For this review, take the finished solid that the model builds, in its own axes (mm). A direction names the side the tool comes from. Give positions to 0.01 mm unless a question says otherwise; leave off trailing zeros. Loops run counter-clockwise (first coordinate to the right, second up) from the corner with the lowest first, then second, coordinate; pieces in that order, holes last. Notation, with made-up numbers: (-34.5, -18) - (23.5, -18) arc R26 ccw to (23.5, 15) - close; hole circle Ø3 at (56.25, 6). An arc over 180 degrees is marked (long way). Answer as CSV lines item,"result".
from build123d import *


with BuildPart() as f2:
    # F2: sweep along a path in F1
    with BuildLine(Plane.XY) as f2_path:
        Line((0, 717.2), (0, 6))
        Line((0, 6), (1631.95, 6))
        Line((1631.95, 6), (1631.95, 717.2))
        Line((1631.95, 717.2), (0, 717.2))
    # F0 (on Right) → F2 (sweep)
    with BuildSketch(Plane.YZ):
        with BuildLine():
            Line((0, -6), (0, -70.7))
            Line((0, -70.7), (6, -70.7))
            Line((6, -70.7), (6, -68))
            Line((6, -68), (4.8, -68))
            Line((4.8, -68), (4.8, -69.5))
            Line((4.8, -69.5), (1.5, -69.5))
            Line((1.5, -69.5), (1.5, -6))
            ThreePointArc((1.5, -6), (2.8180194847, -2.8180194847), (6, -1.5))
            Line((6, -1.5), (8.6, -1.5))
            Line((8.6, -1.5), (8.6, -9.4503759398))
            Line((8.6, -9.4503759398), (6, -12.5))
            Line((6, -12.5), (6, -13.7))
            Line((6, -13.7), (6.5538461538, -13.7))
            Line((6.5538461538, -13.7), (8.6, -11.3))
            Line((8.6, -11.3), (8.6, -13.7))
            Line((8.6, -13.7), (43.1, -13.7))
            Line((43.1, -13.7), (43.1, -12.5))
            Line((43.1, -12.5), (9.8, -12.5))
            Line((9.8, -12.5), (9.8, -4.5))
            Line((9.8, -4.5), (13.5, -4.5))
            Line((13.5, -4.5), (13.5, -3.3))
            Line((13.5, -3.3), (9.8, -3.3))
            Line((9.8, -3.3), (9.8, -1.5))
            Line((9.8, -1.5), (12.2, -1.5))
            Line((12.2, -1.5), (12.2, 0))
            Line((12.2, 0), (6, 0))
            ThreePointArc((6, 0), (1.7573593129, -1.7573593129), (0, -6))
        make_face()
    sweep(path=f2_path.line, transition=Transition.RIGHT)


solid = f2.part
1) Draft analysis for pull direction Z (two halves, no side actions). For faces 3 (the flat face through (827, 0, -38)), 4 (the flat face through (752, 700, -13.7)), 5 (the flat face through (827, 1.5, -38)), state which applies: pulls with the +Z half, pulls with the -Z half, needs draft (parallel to the pull), parting line crosses it, or undercut.
From the geometry:
face 3,"needs draft"
face 4,"pulls with the -Z half"
face 5,"undercut"
2) Insertion check: P1, Ø2.5, axis at y = 459, z = -4.5, coming from the +X side; P2, Ø2, axis at y = 445.5, z = -2.5, coming from the +X side. Each pin has a flat end and moves straight along its axis. Give the tip position at first contact, or say it passes through.
From the geometry:
P1,"stops at x = 1637.94"
P2,"stops at x = 1637.4"
3) Machinability: for faces 1 (the flat face through (1637.95, 367, -38)), 2 (the flat face through (1636.45, 367, -38)), which of the approach directions +Z, -Z, +X, -X, +Y, -Y give a long, thin tool a straight path to every point of the face, cutting with its end or side? Answer none if there is none.
From the geometry:
face 1,"+Z, -Z, +X, +Y, -Y"
face 2,"none"
4) Consider section A-A on z = -53. Write out the cut boundary in (x, y).
From the geometry:
outline,"(-6, 0) - (1637.95, 0) - (1637.95, 723.2) - (-6, 723.2) - close; hole (-4.5, 1.5) - (1636.45, 1.5) - (1636.45, 721.7) - (-4.5, 721.7) - close"
5) Wall thickness on line 1 (X direction, y = 231, z = -5.5); line 2 (Y direction, x = 396, z = -9.5); line 3 (X direction, y = 96, z = -9.5): over which ranges is each line inside the solid? List them lowest first. Write a range as from..to.
From the geometry:
line 1,"x = -5.98..-4.47, 2.6..3.8, 1628.15..1629.35, 1636.42..1637.93"
line 2,"y = 0..1.5, 8.56..9.8, 713.4..714.64, 721.7..723.2"
line 3,"x = -6..-4.5, 2.56..3.8, 1628.15..1629.39, 1636.45..1637.95"
